```python
from build123d import *

# Parameters (mm, degrees)
CYLINDER022_R       = 1.6
CYLINDER022_DEPTH   = 20
ARRAY001007_X_COUNT = 2
ARRAY001007_X_PITCH = 10
ARRAY001007_Y_COUNT = 2
ARRAY001007_Y_PITCH = 10
BOX008_W            = 16
BOX008_H            = 16
BOX008_DEPTH        = 1
FILLET003_R         = 4


with BuildPart() as rod_holder_hole_array001:
    # Cylinder022 → Cylinder022 (new body)
    with BuildSketch(Plane(origin=(3, 3, -6), x_dir=(1, 0, 0), z_dir=(0, 0, 1))):
        Circle(CYLINDER022_R)
    extrude(amount=CYLINDER022_DEPTH)

    # Array001007 X: rod holder hole array001 ×2


with BuildPart() as rod_holder_hole_array001_1:
    add(rod_holder_hole_array001.part)
    with Locations(*[(i * ARRAY001007_X_PITCH, 0, 0) for i in range(1, ARRAY001007_X_COUNT)]):
        add(rod_holder_hole_array001.part)

    # Array001007 Y: rod holder hole array001 ×2


with BuildPart() as rod_holder_hole_array001_2:
    add(rod_holder_hole_array001_1.part)
    with Locations(*[(0, i * ARRAY001007_Y_PITCH, 0) for i in range(1, ARRAY001007_Y_COUNT)]):
        add(rod_holder_hole_array001_1.part)


with BuildPart() as rod_cover_fillet:
    # Box008 → Box008 (new body)
    with BuildSketch(Plane.XY):
        with Locations((8, 8)):
            Rectangle(BOX008_W, BOX008_H)
    extrude(amount=BOX008_DEPTH)

    # Cut006: cut rod holder hole array001
    add(rod_holder_hole_array001_2.part, mode=Mode.SUBTRACT)

    # Fillet003
    fillet003_edges = [rod_cover_fillet.edges().sort_by_distance(p)[0] for p in [
        (0, 0, 0.5),
        (0, 16, 0.5),
        (16, 0, 0.5),
        (16, 16, 0.5),
    ]]
    fillet(fillet003_edges, radius=FILLET003_R)


solid = rod_cover_fillet.part
```
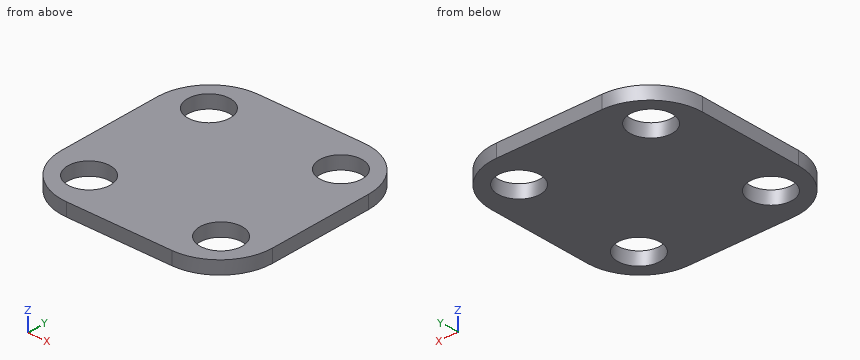
The model under review builds one solid part; all positions refer to its coordinate system, in mm. Round coordinates to 2 decimals unless told otherwise and drop trailing zeros. Loops run counter-clockwise (first coordinate to the right, second up) from the corner with the lowest first, then second, coordinate; pieces in that order, holes last.
1) Wall thickness on line 1 along X through (y, z) = (13, 0.6); line 2 along X through (y, z) = (12.5, 0.15): over which ranges is each line inside the solid? List them lowest first.
Values follow:
line 1: x = 0.13 to 1.4, 4.6 to 11.4, 14.6 to 15.87
line 2: x = 0.03 to 1.48, 4.52 to 11.48, 14.52 to 15.97
2) Consider section B-B on z = 0.35. State the section outline as (x, y) points, then the cut area to 3 significant figures.
Values follow:
outline: (0, 4) arc R4 ccw to (4, 0) - (12, 0) arc R4 ccw to (16, 4) - (16, 12) arc R4 ccw to (12, 16) - (4, 16) arc R4 ccw to (0, 12) - close; hole circle Ø3.2 at (3, 3); hole circle Ø3.2 at (3, 13); hole circle Ø3.2 at (13, 3); hole circle Ø3.2 at (13, 13)
area: 210 mm2
3) Consider section A-A on x = 2.25. State the section outline as (y, z) points, then the cut area to 3 significant figures.
Values follow:
outline: (0.4, 0) - (1.59, 0) - (1.59, 1) - (0.4, 1) - close; (4.41, 0) - (11.59, 0) - (11.59, 1) - (4.41, 1) - close; (14.41, 0) - (15.6, 0) - (15.6, 1) - (14.41, 1) - close
area: 9.54 mm2
